Autodesk Inventor part; units mm, degrees
ref_plane "Arbeitsebene1" through (0, 0, 40) normal (0, 0, 1) x (1, 0, 0)
ref_plane "YZ Plane" through (0, 0, 0) normal (1, 0, 0) x (0, 1, 0)
ref_plane "XZ Plane" through (0, 0, 0) normal (0, 1, 0) x (-1, 0, 0)
sketch "Skizze1" plane through (0, 0, 0) normal (0, 0, 1) x (1, 0, 0)
  line L0 (0, 0) -> (50, 0)
  line L1 (50, 0) -> (50, 12)
  line L2 (50, 12) -> (0, 12)
  line L3 (0, 12) -> (0, 0)
extrude "Extrusion1" add sketch "Skizze1" along normal blind 40
ref_plane "Arbeitsebene1" through (0, 0, 40) normal (0, 0, 1) x (1, 0, 0)
sketch "Skizze2" plane through (0, 0, 40) normal (0, 0, 1) x (1, 0, 0)
  line L0 (29, 0) -> (47, 0)
  line L1 (47, 0) -> (47, 5)
  line L2 (47, 5) -> (29, 5)
  line L3 (29, 5) -> (29, 0)
extrude "Extrusion2" cut sketch "Skizze2" against normal blind 28
sketch "Skizze3" plane through (0, 0, 40) normal (0, 0, 1) x (1, 0, 0)
  line L0 (2, 0) -> (24, 0)
  line L1 (24, 0) -> (24, 6.3)
  line L2 (24, 6.3) -> (2, 6.3)
  line L3 (2, 6.3) -> (2, 0)
extrude "Extrusion3" cut sketch "Skizze3" against normal blind 25
sketch "Skizze4" plane through (0, 0, 0) normal (0, 1, 0) x (-1, 0, 0)
  circle A0 centre (38, 20) radius 2
extrude "Extrusion4" cut sketch "Skizze4" along normal mid plane 30
sketch "Skizze5" plane through (0, 0, 40) normal (0, 0, 1) x (1, 0, 0)
  circle A0 centre (13, 0) radius 2.5
extrude "Extrusion5" cut sketch "Skizze5" against normal blind 5
sketch "Skizze6" plane through (0, 0, 0) normal (0, 0, 1) x (1, 0, 0)
  circle A0 centre (4, -8) radius 2.1
  circle A1 centre (4, 8) radius 2.1
  circle A2 centre (46, -8) radius 2.1
  circle A3 centre (46, 8) radius 2.1
extrude "Extrusion6" cut sketch "Skizze6" along normal blind 5
properties part number "Motorhalterung"
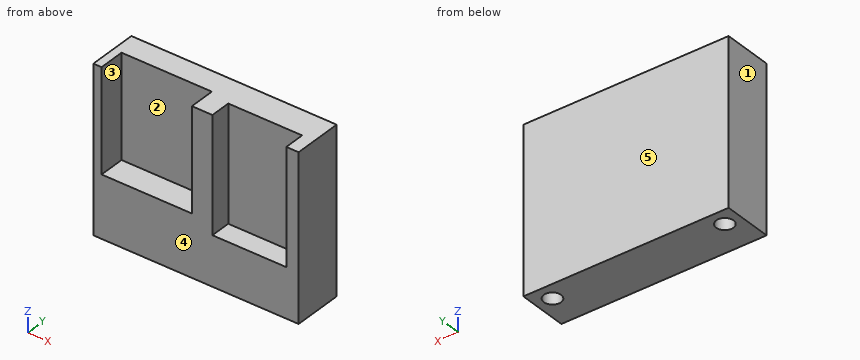
The listing builds one solid part. Answer for the finished solid, in the listing's coordinates (mm). Face numbers are marked on the shaded views. A direction names the side the tool comes from. Give positions to 0.01 mm unless a question says otherwise; leave off trailing zeros. Write each loop counter-clockwise with the first axis right and the second up, starting at its lowest first coordinate (ties: lowest second). Pieces come first, ordered by that corner, then holes.
1) Find the intervals of material crossed by L1, parallel to Y at x = 4, z = 1.5; L2, parallel to Y at x = 38, z = 30.5; L3, parallel to Z at x = 21, y = 6, in increasing order.
2) For a pull along Y with two mould halves and no side action, classify the marked faces 3, 4 and 5 as pulls with the +Y half, pulls with the -Y half, needs draft (parallel to the pull), parting line crosses it, or undercut.
3) Given P1, Ø3.5, axis at x = 46, y = 8, coming from the -Z side; P2, Ø7, axis at x = 14.5, y = 1.5, coming from the +Z side; P3, Ø2.5, axis at x = 42, y = 3, coming from the +Z side, each flat-ended and moving along its own axis, determine where each tip first touches the part or whether it passes through.
4) Section C-C (z = 18) is taken. Write down the section's boundary in (x, y).
5) Section D-D (z = 3) is taken. Write down the section's boundary in (x, y), and give its area (3 significant figures).
6) A tool of negligible diameter and unlimited length cuts with its end or side. For the marked faces 1 and 2, from which of +Z, -Z, +X, -X, +Y, -Y can it reach the whole face along a straight path? Write none if from no direction.
7) Section B-B (x = 4) is taken. Write down the section's boundary in (y, z), and give its area (4 significant figures).
8) Section A-A (y = 8) is taken. Write down the section's boundary in (x, z), and give its area (3 significant figures).
Response:
1. L1: y = 0 to 5.9, 10.1 to 12
1. L2: y = 5 to 12
1. L3: z = 0 to 15
2. face 3: needs draft
2. face 4: pulls with the -Y half
2. face 5: pulls with the +Y half
3. P1: stops at z = 5
3. P2: stops at z = 15
3. P3: stops at z = 12
4. outline: (0, 0) - (2, 0) - (2, 6.3) - (24, 6.3) - (24, 0) - (29, 0) - (29, 5) - (47, 5) - (47, 0) - (50, 0) - (50, 12) - (0, 12) - close
5. outline: (0, 0) - (50, 0) - (50, 12) - (0, 12) - close; hole circle Ø4.2 at (4, 8); hole circle Ø4.2 at (46, 8)
5. area: 572 mm2
6. face 1: +Z, -Z, -X, +Y, -Y
6. face 2: +Z, -Y
7. outline: (0, 0) - (5.9, 0) - (5.9, 5) - (10.1, 5) - (10.1, 0) - (12, 0) - (12, 40) - (6.3, 40) - (6.3, 15) - (0, 15) - close
7. area: 301.5 mm2
8. outline: (0, 0) - (1.9, 0) - (1.9, 5) - (6.1, 5) - (6.1, 0) - (43.9, 0) - (43.9, 5) - (48.1, 5) - (48.1, 0) - (50, 0) - (50, 40) - (0, 40) - close
8. area: 1,960 mm2
